```python
from build123d import *

# Parameters (mm, degrees)
SKETCH1_R           = 2.5
BOSS_EXTRUDE1_DEPTH = 4
SKETCH2_W           = 4
SKETCH2_H           = 22
BOSS_EXTRUDE2_DEPTH = 10
SKETCH3_R           = 2.5
CUT_EXTRUDE1_DEPTH  = 20


with BuildPart() as part:
    # Sketch1 → Boss-Extrude1 (new body)
    with BuildSketch(Plane(origin=(0, 0, 0), x_dir=(1, 0, 0), z_dir=(0, 1, 0))):
        Polygon((32, 60), (80, 12), (80, 0), (0, 0), (0, 60), align=None)
        with Locations(Location((24, 40.35, 0), (0, 0, 270))):
            Circle(SKETCH1_R, mode=Mode.SUBTRACT)
        with Locations(Location((72.5, 7.5, 0), (0, 0, 270))):
            Circle(SKETCH1_R, mode=Mode.SUBTRACT)
    extrude(amount=BOSS_EXTRUDE1_DEPTH)

    # Sketch2 → Boss-Extrude2 (add)
    with BuildSketch(Plane(origin=(0, 4, 0), x_dir=(1, 0, 0), z_dir=(0, 1, 0))):
        with Locations((2, 11)):
            Rectangle(SKETCH2_W, SKETCH2_H)
    extrude(amount=BOSS_EXTRUDE2_DEPTH)

    # Sketch3 → Cut-Extrude1 (cut)
    with BuildSketch(Plane.ZY):
        with Locations((-18, 9)):
            Circle(SKETCH3_R)
        with Locations((-4, 9)):
            Circle(SKETCH3_R)
    extrude(amount=-CUT_EXTRUDE1_DEPTH, mode=Mode.SUBTRACT)


solid = part.part
```
Part model, mm, in its own coordinate system. A direction names the side the tool comes from. Round coordinates to 2 decimals unless told otherwise and drop trailing zeros. Loops run counter-clockwise (first coordinate to the right, second up) from the corner with the lowest first, then second, coordinate; pieces in that order, holes last.
Item 1: Drill centre lines: line 1 (X direction, y = 1.45, z = -7.5); line 2 (Y direction, x = 52.5, z = -13). Where is each one in solid material? Low to high.
Item 2: Drop flat-ended pins along their axis: P1, Ø4, axis at x = 46.5, z = -33.5, coming from the +Y side; P2, Ø4, axis at x = 24, z = -40.35, coming from the -Y side; P3, Ø1, axis at y = 1.5, z = -33, coming from the +X side; P4, Ø1.2, axis at x = 2, y = 10.5, coming from the -Z side. Give the stop position or say it passes through.
Item 3: Mould opens along Z. For faces 1 (the face through (80, 2, -6)), 2 (the face through (70.06, 1.97, -8.04)), 3 (the face through (30.6, 3.8, 0)) say: +Z half, -Z half, draft (parallel to the pull), parting line (faces both ways), or undercut.
Item 4: Cut at C-C, the plane z = -4. Give the cut face in (x, y), then the cut area to 3 significant figures.
Item 5: Cut at B-B, the plane y = 9. Give the cut face in (x, z), then the cut area to 3 significant figures.
Item 6: 3-axis set-ups, long thin cutter, end or side, ignore diameter. For faces 4 (the face through (4, 9, -11)), 5 (the face through (2, 9, -22)), 6 (the face through (24.751, 1.972, -37.965)): which of +Z, -Z, +X, -X, +Y, -Y reach the whole face in a straight line?
Item 7: Cut at A-A, the plane x = 24. Give the cut face in (y, z), then the cut area to 3 significant figures.
Item 8: Cut at D-D, the plane z = -18. Give the cut face in (x, y), then the cut area to 3 significant figures.
A:
1. line 1: x = 0 to 70, 75 to 80
1. line 2: y = 0 to 4
2. P1: stops at y = 4
2. P2: passes through
2. P3: stops at x = 59.5
2. P4: stops at z = -22
3. face 1: draft
3. face 2: undercut
3. face 3: +Z half
4. outline: (0, 0) - (80, 0) - (80, 4) - (4, 4) - (4, 6.5) - (0, 6.5) - close; (0, 11.5) - (4, 11.5) - (4, 14) - (0, 14) - close
4. area: 340 mm2
5. outline: (0, -22) - (4, -22) - (4, -20.5) - (0, -20.5) - close; (0, -15.5) - (4, -15.5) - (4, -6.5) - (0, -6.5) - close; (0, -1.5) - (4, -1.5) - (4, 0) - (0, 0) - close
5. area: 48.0 mm2
6. face 4: +Z, -Z, +X, +Y
6. face 5: -Z, +X, -X, +Y
6. face 6: +Y, -Y
7. outline: (0, -60) - (4, -60) - (4, -42.85) - (0, -42.85) - close; (0, -37.85) - (4, -37.85) - (4, 0) - (0, 0) - close
7. area: 220 mm2
8. outline: (0, 0) - (74, 0) - (74, 4) - (4, 4) - (4, 6.5) - (0, 6.5) - close; (0, 11.5) - (4, 11.5) - (4, 14) - (0, 14) - close
8. area: 316 mm2
